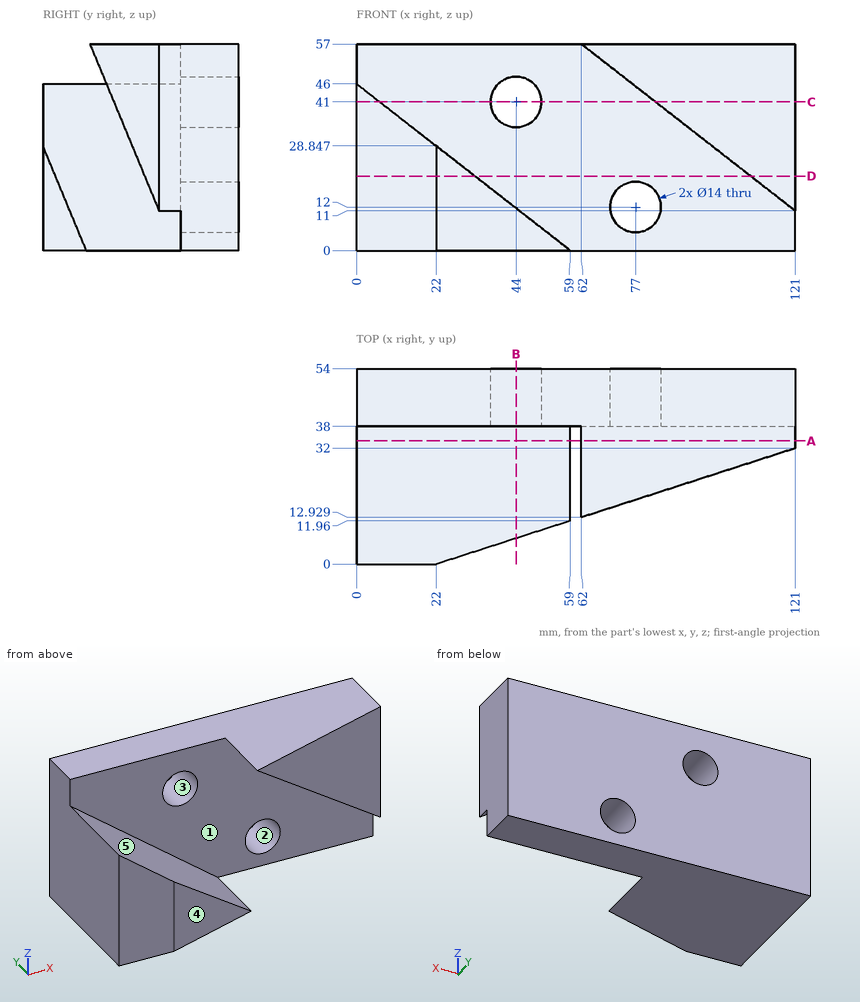
Input: dimensioned drawing with shaded views. Units: mm. Origin: part minimum x, y, z. A direction names the side the tool comes from. Give positions to 0.01 mm unless a question says otherwise; leave off trailing zeros. Write each loop counter-clockwise with the first axis right and the second up, starting at its lowest first coordinate (ties: lowest second). Pieces come first, ordered by that corner, then holes. Notation, with made-up numbers: M -29.5,-4.75 L -13.5,-4.75 A24 ccw -13.5,17.25 Z; hole C 77,71.5 d9. An arc over 180 degrees is marked long. Return JSON: item names as keys, results as strings. Group by question number.
1) Cut plane C-C, the plane z = 41. Output: boundary loops of the cut face in (x, y).
2) Cut plane B-B, the plane x = 44. Output: boundary loops of the cut face in (y, z) (1 decimal), plus the area to 3 significant figures.
3) Set-up query: the marked faces 1 and 2. Return all of +Z, -Z, +X, -X, +Y, -Y with unobstructed straight access to the full face (end or side cutting, diameter ignored); none if empty.
4) Pin query (flat end, axial travel): P1, Ø5, axis at y = 12.5, z = 26.5, coming from the +X side; P2, Ø6, axis at x = 64, y = 22.5, coming from the -Z side; P3, Ø18, axis at x = 77, z = 12, coming from the -Y side. Return the tip coordinate at first contact, or that it passes through.
5) Pull-direction query (Z, two-part tool) for the marked faces 3, 4 and 5; classes: pulls with the +Z half, pulls with the -Z half, needs draft (parallel to the pull), parting line crosses it, or undercut.
6) Material intervals for line 1 along Z through (x, y) = (44, 48); line 2 along Z through (x, y) = (77, 48.5); line 3 along Y through (x, z) = (14.5, 44), sorted ascending. Write a range as [from, to].
7) Cut plane D-D, the plane z = 20.5. Output: boundary loops of the cut face in (x, y) (1 decimal), plus the area to 3 significant figures.
8) Cut plane A-A, the plane y = 34. Output: boundary loops of the cut face in (x, z), plus the area to 3 significant figures.
Recorded:
{
 "1": {"outline": "M 0,0 L 6.41,0 L 6.41,38 L 37,38 L 37,54 L 0,54 Z; M 51,38 L 82.52,38 L 82.52,19.56 L 121,32 L 121,54 L 51,54 Z"},
 "2": {"outline": "M 7.1,0 L 54,0 L 54,34 L 38,34 L 38,11.7 L 7.1,11.7 Z; M 38,48 L 54,48 L 54,57 L 38,57 Z", "area": "1,050 mm²"},
 "3": {"face 1": "-Y", "face 2": "+Y, -Y"},
 "4": {"P1": "stops at x = 28.22", "P2": "stops at z = 53.1", "P3": "stops at y = 38"},
 "5": {"face 3": "undercut", "face 4": "needs draft", "face 5": "pulls with the +Z half"},
 "6": {"line 1": "z = [0, 34], [48, 57]", "line 2": "z = [0, 5], [19, 57]", "line 3": "y = [38, 54]"},
 "7": {"outline": "M 0,0 L 22,0 L 32.7,3.5 L 32.7,38 L 108.8,38 L 108.8,28.1 L 121,32 L 121,54 L 0,54 Z", "area": "3,260 mm²"},
 "8": {"outline": "M 0,0 L 59,0 L 0,46 Z; M 62,57 L 121,11 L 121,57 Z", "area": "2,710 mm²"}
}
